from build123d import *

# Parameters (mm, degrees)
SKETCH1_W             = 18.6
SKETCH1_H             = 26.2
SKETCH1_R             = 1.25
BOSS_EXTRUDE1_DEPTH   = 1.2
SKETCH3_W             = 12.2
SKETCH3_H             = 12
BOSS_EXTRUDE2_DEPTH   = 4.4
SKETCH10_W            = 1.45
SKETCH10_H            = 0.2
SKETCH13_W            = 1.45
SKETCH13_H            = 0.2
LPATTERN1_COUNT       = 2
LPATTERN1_PITCH       = 2.85
LPATTERN2_COUNT       = 2
LPATTERN2_PITCH       = 2.85
SKETCH14_R            = 3.5
BOSS_EXTRUDE4_DEPTH   = 7.1
CHAMFER1_SIZE         = 0.3
SKETCH15_R            = 1.9
BOSS_EXTRUDE5_DEPTH   = 0.65
SKETCH16_R            = 3
BOSS_EXTRUDE6_DEPTH   = 14.45
CHAMFER2_SIZE         = 0.6
CUT_EXTRUDE1_DEPTH    = 10.8
SKETCH18_R            = 0.35
CUT_EXTRUDE2_DEPTH    = 1.2
SKETCH19_W            = 1.5
SKETCH19_H            = 2.5
SKETCH19_R            = 0.35
BOSS_EXTRUDE7_DEPTH   = 0.01
FILLET1_R             = 0.5
CROQUIS1_R            = 3.5
CORTAR_EXTRUIR1_DEPTH = 8.9
REDONDEO1_R           = 0.3


with BuildPart() as part:
    # Sketch1 → Boss-Extrude1 (new body)
    with BuildSketch(Plane(origin=(0, 0, 0), x_dir=(1, 0, 0), z_dir=(0, 1, 0))):
        Rectangle(SKETCH1_W, SKETCH1_H)
        with Locations((-7.3, 8.3)):
            Circle(SKETCH1_R, mode=Mode.SUBTRACT)
        with Locations((-7.3, -5.4)):
            Circle(SKETCH1_R, mode=Mode.SUBTRACT)
    extrude(amount=BOSS_EXTRUDE1_DEPTH)

    # Sketch3 → Boss-Extrude2 (add)
    with BuildSketch(Plane(origin=(0, 1.2, 0), x_dir=(1, 0, 0), z_dir=(0, 1, 0))):
        with Locations((1.1, 2.8)):
            Rectangle(SKETCH3_W, SKETCH3_H)
    extrude(amount=BOSS_EXTRUDE2_DEPTH)

    # Sweep3: sweep along a curve in space
    with BuildLine() as sweep3_path:
        Line((-1.325, 2.85, 3.2), (-1.325, 2.85, 4.3))
        ThreePointArc((-1.325, 2.85, 4.3), (-1.325, 2.703553391, 4.653553391), (-1.325, 2.35, 4.8))
        Line((-1.325, 2.35, 4.8), (-1.325, 1.2, 4.8))
    # Sketch10 → Sweep3 (sweep)
    with BuildSketch(Plane.XY.offset(3.2)):
        with Locations((-1.325, 2.85)):
            Rectangle(SKETCH10_W, SKETCH10_H)
    sweep3 = sweep(path=sweep3_path.line)

    # Mirror2: Sweep3 across plane
    add(sweep3.mirror(Plane.ZY.offset(-1.1)))

    # Sweep4: sweep along a curve in space
    with BuildLine() as sweep4_path:
        Line((1.1, 2.8, -8.8), (1.1, 2.8, -9.75))
        ThreePointArc((1.1, 2.8, -9.75), (1.1, 2.653553391, -10.103553391), (1.1, 2.3, -10.25))
        Line((1.1, 2.3, -10.25), (1.1, 1.2, -10.25))
    # Sketch13 → Sweep4 (sweep)
    with BuildSketch(Plane(origin=(0, 0, -8.8), x_dir=(-1, 0, 0), z_dir=(0, 0, -1))):
        with Locations((-1.1, 2.8)):
            Rectangle(SKETCH13_W, SKETCH13_H)
    sweep4 = sweep(path=sweep4_path.line)

    # LPattern1: Sweep4 ×2
    with Locations(*[(-i * LPATTERN1_PITCH, 0, 0) for i in range(1, LPATTERN1_COUNT)]):
        add(sweep4)

    # LPattern2: Sweep4 ×2
    with Locations(*[(i * LPATTERN2_PITCH, 0, 0) for i in range(1, LPATTERN2_COUNT)]):
        add(sweep4)

    # Sketch14 → Boss-Extrude4 (add)
    with BuildSketch(Plane(origin=(0, 5.6, 0), x_dir=(1, 0, 0), z_dir=(0, 1, 0))):
        with Locations((1.1, 2.8)):
            Circle(SKETCH14_R)
    extrude(amount=BOSS_EXTRUDE4_DEPTH)

    # Chamfer1
    chamfer1_edges = [part.edges().sort_by_distance(p)[0] for p in [
        (-2.4, 12.7, -2.8),
    ]]
    chamfer(chamfer1_edges, length=CHAMFER1_SIZE)

    # Sketch15 → Boss-Extrude5 (add)
    with BuildSketch(Plane(origin=(0, 12.7, 0), x_dir=(1, 0, 0), z_dir=(0, 1, 0))):
        with Locations((1.1, 2.8)):
            Circle(SKETCH15_R)
    extrude(amount=BOSS_EXTRUDE5_DEPTH)

    # Sketch16 → Boss-Extrude6 (add)
    with BuildSketch(Plane(origin=(0, 13.35, 0), x_dir=(1, 0, 0), z_dir=(0, 1, 0))):
        with Locations((1.1, 2.8)):
            Circle(SKETCH16_R)
    extrude(amount=BOSS_EXTRUDE6_DEPTH)

    # Chamfer2
    chamfer2_edges = [part.edges().sort_by_distance(p)[0] for p in [
        (-1.9, 27.8, -2.8),
    ]]
    chamfer(chamfer2_edges, length=CHAMFER2_SIZE)

    # Sketch17 → Cut-Extrude1 (cut)
    with BuildSketch(Plane(origin=(0, 27.8, 0), x_dir=(1, 0, 0), z_dir=(0, 1, 0))):
        with BuildLine():
            Line((-0.396662955, 5.4), (-0.396662955, 0.2))
            ThreePointArc((-0.396662955, 0.2), (-1.9, 2.8), (-0.396662955, 5.4))
        make_face()
    extrude(amount=-CUT_EXTRUDE1_DEPTH, mode=Mode.SUBTRACT)

    # Sketch18 → Cut-Extrude2 (cut)
    with BuildSketch(Plane(origin=(0, 1.2, 0), x_dir=(1, 0, 0), z_dir=(0, 1, 0))):
        with Locations((6.5, -11)):
            Circle(SKETCH18_R)
        with Locations((3.96, -11)):
            Circle(SKETCH18_R)
        with Locations((1.42, -11)):
            Circle(SKETCH18_R)
        with Locations((-1.12, -11)):
            Circle(SKETCH18_R)
        with Locations((-3.66, -11)):
            Circle(SKETCH18_R)
    extrude(amount=-CUT_EXTRUDE2_DEPTH, mode=Mode.SUBTRACT)

    # Sketch19 → Boss-Extrude7 (add)
    with BuildSketch(Plane(origin=(0, 1.2, 0), x_dir=(1, 0, 0), z_dir=(0, 1, 0))):
        with Locations((3.96, -11)):
            Rectangle(SKETCH19_W, SKETCH19_H)
        with Locations((3.96, -11)):
            Circle(SKETCH19_R, mode=Mode.SUBTRACT)
        with Locations((6.5, -11)):
            Rectangle(SKETCH19_W, SKETCH19_H)
        with Locations((6.5, -11)):
            Circle(SKETCH19_R, mode=Mode.SUBTRACT)
        with Locations((1.42, -11)):
            Rectangle(SKETCH19_W, SKETCH19_H)
        with Locations((1.42, -11)):
            Circle(SKETCH19_R, mode=Mode.SUBTRACT)
        with Locations((-1.12, -11)):
            Rectangle(SKETCH19_W, SKETCH19_H)
        with Locations((-1.12, -11)):
            Circle(SKETCH19_R, mode=Mode.SUBTRACT)
        with Locations((-3.66, -11)):
            Rectangle(SKETCH19_W, SKETCH19_H)
        with Locations((-3.66, -11)):
            Circle(SKETCH19_R, mode=Mode.SUBTRACT)
    boss_extrude7 = extrude(amount=BOSS_EXTRUDE7_DEPTH)

    # Mirror3: Boss-Extrude7 across plane
    add(boss_extrude7.mirror(Plane.ZX.offset(0.6)))

    # Fillet1
    fillet1_edges = [part.edges().sort_by_distance(p)[0] for p in [
        (7.2, 3.4, 3.2),
        (7.2, 3.4, -8.8),
        (-5, 3.4, -8.8),
        (-5, 3.4, 3.2),
    ]]
    fillet(fillet1_edges, radius=FILLET1_R)

    # Croquis1 → Cortar-Extruir1 (cut)
    with BuildSketch(Plane(origin=(0, 27.8, 0), x_dir=(1, 0, 0), z_dir=(0, 1, 0))):
        with Locations((1.1, 2.8)):
            Circle(CROQUIS1_R)
    extrude(amount=-CORTAR_EXTRUIR1_DEPTH, mode=Mode.SUBTRACT)

    # Redondeo1
    redondeo1_edges = [part.edges().sort_by_distance(p)[0] for p in [
        (2.601667596, 18.9, -5.397112711),
    ]]
    fillet(redondeo1_edges, radius=REDONDEO1_R)


solid = part.part
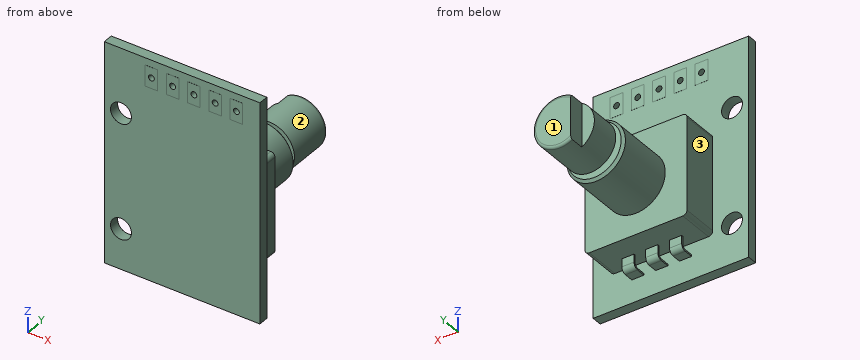
Geometry: final body of the model. Coordinates: model frame, mm. Face numbers are marked on the shaded views. A direction names the side the tool comes from. Give positions to 0.01 mm unless a question says otherwise; leave off trailing zeros. Write each loop counter-clockwise with the first axis right and the second up, starting at its lowest first coordinate (ties: lowest second). Pieces come first, ordered by that corner, then holes. Notation, with made-up numbers: M 38.25,61.25 L 82.25,61.25 A27 ccw 82.25,78.25 Z; hole C 38.25,17.5 d5. An arc over 180 degrees is marked long. Answer in a Markdown table with one row per item. Add a question column.
(1) Section A-A on x = -6.75. Return loops of the section in (y, z), and give its area (3 significant figures).
(2) Ray query, line 1 (Z direction, x = -7.3, y = 0.55); line 2 (X direction, y = 0.95, z = 11); line 3 (X direction, y = 1, z = 10.75). Return the intervals inside material, ascending.
(3) Section C-C on y = 9.25. Return loops of the section in (x, z), and give its area (3 significant figures).
(4) Reachability of the marked faces 1, 2 and 3 from +Z, -Z, +X, -X, +Y, -Y: full face, straight path, thin tool, end or side. Return the list, or none.
(5) Section D-D on y = 15. Return loops of the section in (x, z).
(6) Section B-B on z = 11. State how many separate pieces and enclosed holes the cut face has, and give its area (3 significant figures).
(7) First-contact query: pin 1 (6 mm diameter, centred on x = -7, z = -5, fed in from +Y); pin 2 (1.2 mm diameter, centred on x = 3.5, z = 3.5, fed in from -Y); pin 3 (8 mm diameter, centred on y = 12, z = 7, fed in from +X); pin 4 (1.5 mm diameter, centred on x = 0, z = 10, fed in from +Y). Flat tips, straight axial feed; report the tip coordinate or a pass-through.
Result set:
| question | item | result |
|---|---|---|
| 1 | outline | M 0,-13.1 L 1.2,-13.1 L 1.2,-9.42 L 0,-9.42 Z; M 0,-7.18 L 1.2,-7.18 L 1.2,4.28 L 0,4.28 Z; M 0,6.52 L 1.2,6.52 L 1.2,13.1 L 0,13.1 Z |
| 1 | area | 26.1 mm^2 |
| 2 | line 1 | z = -13.1 to -9.55, -7.05 to 4.15, 6.65 to 13.1 |
| 2 | line 2 | x = -9.3 to -4.01, -3.31 to -1.47, -0.77 to 1.07, 1.77 to 3.61, 4.31 to 6.15, 6.85 to 9.3 |
| 2 | line 3 | x = -9.3 to -3.9, -3.42 to -1.36, -0.88 to 1.18, 1.66 to 3.72, 4.2 to 6.26, 6.74 to 9.3 |
| 3 | outline | C 1.1,-2.8 d7 |
| 3 | area | 38.5 mm^2 |
| 4 | face 1 | +Z, -Z, +X, -X, +Y |
| 4 | face 2 | +Y |
| 4 | face 3 | +Z, -Z, -X, +Y |
| 5 | outline | C 1.1,-2.8 d6 |
| 6 | separate pieces | 6 |
| 6 | enclosed holes | 0 |
| 6 | area | 18.2 mm^2 |
| 7 | pin 1 | stops at y = 5.6 |
| 7 | pin 2 | stops at y = 0 |
| 7 | pin 3 | passes through |
| 7 | pin 4 | stops at y = 1.21 |
